from build123d import *

# Parameters (mm, degrees)
F0_W      = 50
F0_H      = 25
F1_DEPTH  = 12.5
F2_R      = 3.5
F3_DEPTH  = 5
F4_SIZE   = 10
F5_SIZE   = 3
F6_W      = 2.1288916469
F6_H      = 25
F7_DEPTH  = 2
F8_W      = 9.6029471606
F8_H      = 18.9187433571
F9_DEPTH  = 1
F10_W     = 13.8777932152
F10_H     = 7.1009902749
F10_W_2   = 21.5250877663
F10_H_2   = 7.2504867127
F11_DEPTH = 3
F12_W     = 6.9172445219
F12_H     = 21.7759581094
F13_DEPTH = 1
F14_W     = 2.5
F14_H     = 4
F15_DEPTH = 2
F16_W     = 2.5
F16_H     = 5
F17_DEPTH = 2


# Not quite as in the source:
# - a pattern or mirror of a feature is missing from the dataset's text; its kind, count and spacing are read off the source's solid


with BuildPart() as f1:
    # F0 (on Top) → F1 (new body, symmetric)
    with BuildSketch(Plane.XY):
        with Locations((1.3995850459, -7.8662077549)):
            Rectangle(F0_W, F0_H)
    extrude(amount=F1_DEPTH, both=True)

    # F2 (on face) → F3 (cut)
    with BuildSketch(Plane.XY.offset(12.5)):
        with Locations((-11.2899886444, -20.3662077549)):
            Circle(F2_R)
        with Locations((8.1175947562, -20.3662077549)):
            Circle(F2_R)
        with Locations((18.194610253, -20.3662077549)):
            Circle(F2_R)
    f3 = extrude(amount=-F3_DEPTH, mode=Mode.SUBTRACT)

    # F3_copies: F3 across plane
    add(f3.mirror(Plane(origin=(0, 0, 0), x_dir=(-1, 0, 0), z_dir=(0, 0, -1))), mode=Mode.SUBTRACT)

    # F4
    f4_edges = [f1.edges().sort_by_distance(p)[0] for p in [
        (-23.600415, 4.633792, 0),
    ]]
    chamfer(f4_edges, length=F4_SIZE)

    # F5
    f5_edges = [f1.edges().sort_by_distance(p)[0] for p in [
        (26.399585, -20.366208, 0),
    ]]
    chamfer(f5_edges, length=F5_SIZE)

    # F6 (on face) → F7 (join)
    with BuildSketch(Plane(origin=(-23.6004149541, 0, 0), x_dir=(0, -1, 0), z_dir=(-1, 0, 0))):
        with Locations((17.0801598579, 0)):
            Rectangle(F6_W, F6_H)
    extrude(amount=F7_DEPTH)

    # F8 (on face) → F9 (cut, symmetric)
    with BuildSketch(Plane(origin=(-9.1171035996, 9.1171035996, 0), x_dir=(-0.7071067812, -0.7071067812, 0), z_dir=(-0.7071067812, 0.7071067812, 0))):
        with Locations((13.4759480134, -0.2812528983)):
            Rectangle(F8_W, F8_H)
    extrude(amount=F9_DEPTH, both=True, mode=Mode.SUBTRACT)

    # F10 (on face) → F11 (cut)
    with BuildSketch(Plane.XY.offset(12.5)):
        with Locations((-6.9388966076, -1.3492055004)):
            Rectangle(F10_W, F10_H)
        Polygon((-13.8777932152, -4.8997006379), (-13.8777932152, 2.201289637), (-20.6305080792, -4.551425227), align=None)
        with Locations((13.1223001517, -1.7409643986)):
            Rectangle(F10_W_2, F10_H_2)
    f11 = extrude(amount=-F11_DEPTH, mode=Mode.SUBTRACT)

    # F11_copies: F11 across plane
    add(f11.mirror(Plane(origin=(0, 0, 0), x_dir=(-1, 0, 0), z_dir=(0, 0, -1))), mode=Mode.SUBTRACT)

    # F12 (on face) → F13 (cut, symmetric)
    with BuildSketch(Plane.YZ.offset(26.3995850459)):
        with Locations((-1.2673075544, -2.09453e-05)):
            Rectangle(F12_W, F12_H)
    extrude(amount=F13_DEPTH, both=True, mode=Mode.SUBTRACT)

    # F14 (on face) → F15 (cut)
    with BuildSketch(Plane.YZ.offset(26.3995850459)):
        with Locations((-14.6162077549, -9)):
            Rectangle(F14_W, F14_H)
        with Locations((-14.6162077549, 9)):
            Rectangle(F14_W, F14_H)
    extrude(amount=-F15_DEPTH, mode=Mode.SUBTRACT)

    # F16 (on face) → F17 (cut)
    with BuildSketch(Plane(origin=(-23.6004149541, 0, 0), x_dir=(0, -1, 0), z_dir=(-1, 0, 0))):
        with Locations((13.2657140344, 8.25)):
            Rectangle(F16_W, F16_H)
        with Locations((13.2657140344, -8.25)):
            Rectangle(F16_W, F16_H)
    extrude(amount=-F17_DEPTH, mode=Mode.SUBTRACT)


solid = f1.part
Verification items for the finished model (mm, model axes). A direction names the side the tool comes from. Give positions to 0.01 mm unless a question says otherwise; leave off trailing zeros. Write each loop counter-clockwise with the first axis right and the second up, starting at its lowest first coordinate (ties: lowest second). Pieces come first, ordered by that corner, then holes.
(1) Cross-section at C-C (x = -19). Enter the section's corners in (y, z).
(2) Cross-section at A-A (z = 3). Enter the section's corners in (x, y).
(3) Material ranges on line 1 (Y direction, x = 23, z = 11.75); line 2 (X direction, y = -3.25, z = 11.25); line 3 (X direction, y = -6.75, z = -3.75), recorded low to high.
(4) Gauge pin test, flat ends, axial feed: pin 1 (0.8 mm diameter, centred on y = -13.5, z = -9, fed in from -X); pin 2 (8 mm diameter, centred on x = 18, y = -1, fed in from +Z); pin 3 (1.6 mm diameter, centred on x = 25.5, z = 9, fed in from -Y); pin 4 (2 mm diameter, centred on x = 7, y = 0.5, fed in from +Z). Record the tip position at first contact, or that the pin passes through.
(5) Mould release check, pull along X, two halves, no side actions. Record for faces 5 (the face through (0, -1, -11)), 6 (the face through (-25.6, -17, 0)), 7 (the face through (-25, -18.145, 0)): +X half, -X half, draft (parallel to the pull), parting line (faces both ways), or undercut.
(6) Access from +Z, -Z, +X, -X, +Y, -Y to the whole of each face (thin tool, end or side, straight path). Record for faces 1 (the face through (2.36, -2, -11)), 2 (the face through (23.885, -2, 11)), 3 (the face through (24.4, -15, 9)), 4 (the face through (8.195, -16.867, -10.035)).
(7) Cross-section at B-B (y = -15.25). Enter the section's corners in (x, z), plus the area to 3 significant figures.
(8) Cross-section at D-D (y = -3). Enter the section's corners in (x, z).
Worked out:
1. outline: (-20.37, -12.5) - (-4.64, -12.5) - (-4.64, -9.5) - (-2.92, -9.5) - (-2.92, -12.5) - (-0.77, -12.5) - (-0.77, -9.74) - (-2.18, -9.74) - (-2.18, 9.18) - (-0.77, 9.18) - (-0.77, 12.5) - (-2.92, 12.5) - (-2.92, 9.5) - (-4.64, 9.5) - (-4.64, 12.5) - (-20.37, 12.5) - close
2. outline: (-25.6, -18.14) - (-23.6, -18.14) - (-23.6, -20.37) - (23.4, -20.37) - (26.4, -17.37) - (26.4, -4.73) - (25.4, -4.73) - (25.4, 2.19) - (26.4, 2.19) - (26.4, 4.63) - (-13.6, 4.63) - (-15.25, 2.98) - (-14.54, 2.28) - (-21.33, -4.51) - (-22.04, -3.81) - (-23.6, -5.37) - (-23.6, -16.02) - (-25.6, -16.02) - close
3. line 1: y = -20.37 to -5.37, 1.88 to 4.63
3. line 2: x = -21.48 to -19.33, 0 to 2.36, 23.88 to 26.4
3. line 3: x = -23.6 to 26.4
4. pin 1: stops at x = -21.6
4. pin 2: stops at z = 12.5
4. pin 3: stops at y = -19.07
4. pin 4: stops at z = 9.5
5. face 5: undercut
5. face 6: -X half
5. face 7: draft
6. face 1: -Z
6. face 2: +Z
6. face 3: +X
6. face 4: -Z, -Y
7. outline: (-23.6, -12.5) - (26.4, -12.5) - (26.4, -11) - (24.4, -11) - (24.4, -7) - (26.4, -7) - (26.4, 7) - (24.4, 7) - (24.4, 11) - (26.4, 11) - (26.4, 12.5) - (-23.6, 12.5) - close
7. area: 1,230 mm2
8. outline: (-21.23, -12.5) - (-19.08, -12.5) - (-19.08, -9.5) - (0, -9.5) - (0, -12.5) - (2.36, -12.5) - (2.36, -9.5) - (23.88, -9.5) - (23.88, -12.5) - (26.4, -12.5) - (26.4, -10.89) - (25.4, -10.89) - (25.4, 10.89) - (26.4, 10.89) - (26.4, 12.5) - (23.88, 12.5) - (23.88, 9.5) - (2.36, 9.5) - (2.36, 12.5) - (0, 12.5) - (0, 9.5) - (-19.08, 9.5) - (-19.08, 12.5) - (-21.23, 12.5) - (-21.23, 9.18) - (-19.82, 9.18) - (-19.82, -9.74) - (-21.23, -9.74) - close
